from build123d import *

# Parameters (mm, degrees)
ESBO_O1_R                = 2.1
RESSALTO_EXTRUS_O1_DEPTH = 9.5


with BuildPart() as part:
    # Esboço1 → Ressalto-extrusão1 (new body)
    with BuildSketch(Plane.XY.offset(9.5)):
        with BuildLine():
            Line((-77.652318909, -56.622659468), (-77.652318909, -20.044841126))
            ThreePointArc((-77.652318909, -20.044841126), (-83.652318909, -14.044841126), (-89.652318909, -20.044841126))
            Line((-89.652318909, -20.044841126), (-89.652318909, -56.622659468))
            ThreePointArc((-89.652318909, -56.622659468), (-83.652318909, -62.622659468), (-77.652318909, -56.622659468))
        make_face()
        with Locations((-83.652318909, -56.622659468)):
            Circle(ESBO_O1_R, mode=Mode.SUBTRACT)
        with Locations((-83.652318909, -20.044841126)):
            Circle(ESBO_O1_R, mode=Mode.SUBTRACT)
    extrude(amount=-RESSALTO_EXTRUS_O1_DEPTH)


solid = part.part
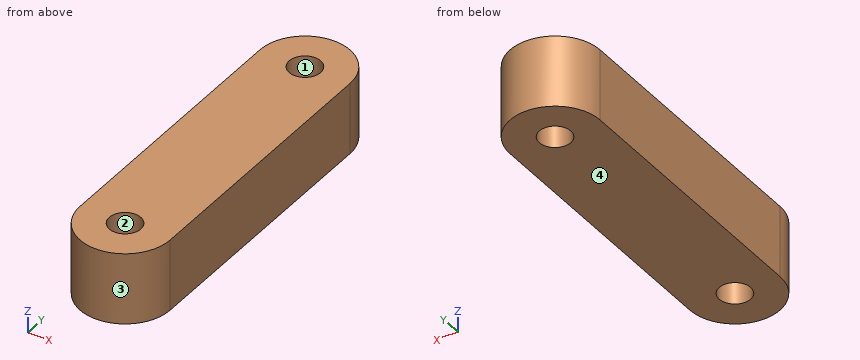
Input: part model. Units: mm. Frame: model coordinates. Face numbers are marked on the shaded views. Coordinates: 2 decimals unless noted, no trailing zeros. Loops run counter-clockwise (first coordinate to the right, second up) from the corner with the lowest first, then second, coordinate; pieces in that order, holes last.
Q1. Cut plane D-D (x = -79.5). Output: boundary loops of the cut face in (y, z).
Q2. Draft query along X for the marked faces 1, 2, 3 and 4. Return one class per face: +X half, -X half, draft (parallel to the pull), parting line (faces both ways), or undercut.
Q3. Cut plane B-B (z = 6.25). Output: boundary loops of the cut face in (x, y), then the cut area to 3 significant figures.
Q4. Cut plane A-A (x = -82.5). Output: boundary loops of the cut face in (y, z), then the cut area to 3 significant figures.
Q5. Cut plane C-C (x = -86.5). Output: boundary loops of the cut face in (y, z).
Q6. Material intervals for line 1 (Y direction, x = -83.5, z = 6.5); line 2 (X direction, y = -20, z = 1.5); line 3 (Y direction, x = -84, z = 1.5), sorted ascending.
Q7. Contact query for flat-ended pins moving along their axis: pin 1 (2 mm diameter, centred on x = -80.5, z = 5.5, fed in from +Y); pin 2 (1.5 mm diameter, centred on x = -81, z = 6, fed in from -Y). Output: stop coordinate, or through.
Working result:
1. outline: (-60.95, 0) - (-15.71, 0) - (-15.71, 9.5) - (-60.95, 9.5) - close
2. face 1: undercut
2. face 2: undercut
2. face 3: parting line
2. face 4: draft
3. outline: (-89.65, -56.62) arc R6 ccw to (-77.65, -56.62) - (-77.65, -20.04) arc R6 ccw to (-89.65, -20.04) - close; hole circle Ø4.2 at (-83.65, -56.62); hole circle Ø4.2 at (-83.65, -20.04)
3. area: 524 mm2
4. outline: (-62.51, 0) - (-58.38, 0) - (-58.38, 9.5) - (-62.51, 9.5) - close; (-54.87, 0) - (-21.8, 0) - (-21.8, 9.5) - (-54.87, 9.5) - close; (-18.29, 0) - (-14.16, 0) - (-14.16, 9.5) - (-18.29, 9.5) - close
4. area: 393 mm2
5. outline: (-61.9, 0) - (-14.76, 0) - (-14.76, 9.5) - (-61.9, 9.5) - close
6. line 1: y = -62.62 to -58.72, -54.53 to -22.14, -17.95 to -14.05
6. line 2: x = -89.65 to -85.75, -81.55 to -77.65
6. line 3: y = -62.61 to -58.69, -54.55 to -22.12, -17.97 to -14.05
7. pin 1: stops at y = -14.44
7. pin 2: stops at y = -62.31
